```python
from build123d import *

# Parameters (mm, degrees)
F2_DEPTH = 25
F3_COUNT = 3
F4_DEPTH = 3
F6_R     = 4.225
F6_R_2   = 2.625
F7_DEPTH = 10
F9_DEPTH = 6
F10_R    = 0.7


# Not quite as in the source:
# - a fillet or chamfer that OpenCascade refuses, or shapes differently, is made with other operations: its cross-section is extruded or revolved along the edge and cut away or added


with BuildPart() as f2:
    # F1 (on Front) → F2 (new body)
    with BuildSketch(Plane.XZ):
        with BuildLine():
            ThreePointArc((0, 1.2), (-0.8485281374, -0.8485281374), (1.2, 0))
            ThreePointArc((1.2, 0), (0.8485281374, 0.8485281374), (0, 1.2))
        make_face()
    extrude(amount=F2_DEPTH)

    # F3: F2 ×3 about axis
    f3_axis = Axis((0, 0, 16.2680745125), (0, 0, 1))


with BuildPart() as f2_1:
    add(f2.part)
    for i in range(1, F3_COUNT):
        add(f2.part.rotate(f3_axis, i * 360 / F3_COUNT))


with BuildPart() as f4:
    # F0 (on Top) → F4 (new body, symmetric)
    with BuildSketch(Plane.XY):
        with BuildLine():
            Line((0, 0), (7.5, 12.9903810568))
            ThreePointArc((7.5, 12.9903810568), (-7.5, 12.9903810568), (-15, 0))
            Line((-15, 0), (0, 0))
        make_face()
        with BuildLine():
            ThreePointArc((-15, 0), (-7.5, -12.9903810568), (7.5, -12.9903810568))
            Line((7.5, -12.9903810568), (0, 0))
            Line((0, 0), (-15, 0))
        make_face()
        with BuildLine():
            ThreePointArc((7.5, -12.9903810568), (12.9903810568, -7.5), (15, 0))
            ThreePointArc((15, 0), (12.9903810568, 7.5), (7.5, 12.9903810568))
            Line((7.5, 12.9903810568), (0, 0))
            Line((0, 0), (7.5, -12.9903810568))
        make_face()
        with BuildLine():
            Line((0, 0), (7.5, 12.9903810568))
            ThreePointArc((7.5, 12.9903810568), (-7.5, 12.9903810568), (-15, 0))
            Line((-15, 0), (0, 0))
        make_face()
        with BuildLine():
            ThreePointArc((-15, 0), (-7.5, -12.9903810568), (7.5, -12.9903810568))
            Line((7.5, -12.9903810568), (0, 0))
            Line((0, 0), (-15, 0))
        make_face()
        with BuildLine():
            ThreePointArc((7.5, -12.9903810568), (12.9903810568, -7.5), (15, 0))
            ThreePointArc((15, 0), (12.9903810568, 7.5), (7.5, 12.9903810568))
            Line((7.5, 12.9903810568), (0, 0))
            Line((0, 0), (7.5, -12.9903810568))
        make_face()
    extrude(amount=F4_DEPTH, both=True)

    # F5: cut F2
    add(f2_1.part, mode=Mode.SUBTRACT)

    # F6 (on face) → F7 (join)
    with BuildSketch(Plane.XY.offset(3)):
        Circle(F6_R)
        Circle(F6_R_2, mode=Mode.SUBTRACT)
    extrude(amount=F7_DEPTH)

    # F8: chamfer of 1 on 2 edges, made by hand

    # F8_s1 → F8_t2 (revolve, cut)
    with BuildSketch(Plane.XZ):
        Polygon((-15, 2), (-14, 3), (-15, 3), align=None)
    revolve(axis=Axis((0, 0, 3), (0, 0, 1)), mode=Mode.SUBTRACT)

    # F8_s3 → F8_t4 (revolve, cut)
    with BuildSketch(Plane.XZ):
        Polygon((-15, -2), (-14, -3), (-15, -3), align=None)
    revolve(axis=Axis((0, 0, -3), (0, 0, 1)), mode=Mode.SUBTRACT)

    # F9 (add): a face of the model
    f9_faces = [f4.faces().sort_by_distance(p)[0] for p in [
        (0, 0, 3),
    ]]
    extrude(f9_faces, amount=-F9_DEPTH)

    # F10
    f10_edges = [f4.edges().sort_by_distance(p)[0] for p in [
        (-2.625, 0, 13),
        (-4.225, 0, 13),
    ]]
    fillet(f10_edges, radius=F10_R)


solid = f4.part
```
Geometry check sheet. Reference: the model listing, model coordinates, mm. A direction names the side the tool comes from. Round coordinates to 2 decimals unless told otherwise and drop trailing zeros. Loops run counter-clockwise (first coordinate to the right, second up) from the corner with the lowest first, then second, coordinate; pieces in that order, holes last. Notation, with made-up numbers: (17, 31.5) - (73, 31.5) arc R32 cw to (73, 68.5) - close; hole circle Ø6 at (68.25, 30). An arc over 180 degrees is marked (long way). Write each question's results on one line, items separated by ' | '. Start each with the question number.
Q1. Release check for a two-part mould opening along Y. For faces 3 (the cylindrical face through (2.5, 0.8, 7.6)), 4 (the flat face through (-3.3, -2.9, 3)), 5 (the cylindrical face through (4.03, 1.27, 7.58)) record: +Y half, -Y half, draft (parallel to the pull), parting line (faces both ways), or undercut.
Q2. Access from +Z, -Z, +X, -X, +Y, -Y to the whole of each face (thin tool, end or side, straight path). Record for faces 1 (the flat face through (0, 0, 3)), 2 (the cylindrical face through (-2.265, 1.328, 0.017)).
Q3. Thickness scan on line 1 (Y direction, x = 0, z = 7.25) (3 decimals); line 2 (Z direction, x = 0, y = -6); line 3 (X direction, y = 2, z = -0.5). Record the ranges inside material, lowest first. Write a range as [from, to].
Q4. Gauge pin test, flat ends, axial feed: P1, Ø8, axis at y = 6, z = 10.5, coming from the -X side; P2, Ø1.5, axis at x = 11, y = 7, coming from the +Z side; P3, Ø5, axis at y = -7, z = 3.5, coming from the +X side. Record the tip position at first contact, or that the pin passes through.
Q5. Cross-section at A-A on z = 6.5. Enter the section's corners in (x, y) (3 decimals).
Answers below:
1) face 3: undercut | face 4: draft | face 5: parting line
2) face 1: +Z | face 2: none
3) line 1: y = [-4.225, -2.625], [2.625, 4.225] | line 2: z = [-3, -1.2], [1.2, 3] | line 3: x = [-14.87, -5.65], [-1.7, 1.7], [5.65, 14.87]
4) P1: stops at x = -3.72 | P2: stops at z = 3 | P3: stops at x = 14.14
5) outline: circle Ø8.45 at (0, 0); hole circle Ø5.25 at (0, 0)
